Verification items for the finished model (mm, model axes). A direction names the side the tool comes from. Round coordinates to 2 decimals unless told otherwise and drop trailing zeros. Write each loop counter-clockwise with the first axis right and the second up, starting at its lowest first coordinate (ties: lowest second). Pieces come first, ordered by that corner, then holes. Notation, with made-up numbers: M -26.5,31 L -2.5,31 A31 ccw -2.5,61 Z; hole C -29,83.5 d8. An arc over 180 degrees is marked long. One line per question, with ' | ' between items. Start each with the question number.
Q1. Release check for a two-part mould opening along X. For faces 5 (the face through (-8, 0.25, 6)), 6 (the face through (2.8, -0.25, 17.4)), 7 (the face through (-4.124, 3.861, 6.522)), 8 (the face through (4.89, 1.06, 13.24)) record: released by +X, released by -X, zero draft, split by the parting line, or undercut.
Q2. Tool access check on faces 1 (the face through (-6, -3.75, 6)), 2 (the face through (-8, 3.25, 7)), 3 (the face through (-7.874, 2.949, 0.285)), 4 (the face through (-8, -2.4, 6)). Record the directions out of +Z, -Z, +X, -X, +Y, -Y that give a thin tool (end or side, any length) a straight path to the whole face; none if there is none.
Q3. Thickness scan on line 1 along Z through (x, y) = (3.5, 3.1); line 2 along Z through (x, y) = (-6.1, -3); line 3 along X through (y, z) = (-2, 15.7). Record the ranges inside material, lowest first. Write a range as from..to.
Q4. Gauge pin test, flat ends, axial feed: pin 1 (5 mm diameter, centred on x = 6, z = 3, fed in from +Y); pin 2 (5.5 mm diameter, centred on y = 3, z = 17, fed in from -X); pin 3 (0.9 mm diameter, centred on x = 4, z = 15.5, fed in from -Y). Record the tip position at first contact, or that the pin passes through.
Q5. Cross-section at B-B (z = 15). Record the boundary of the cut face in (x, y) (3 decimals).
Q6. Cross-section at C-C (x = -7). Record the boundary of the cut face in (y, z) (3 decimals), then the cut area to 3 significant figures.
Q7. Cross-section at A-A (y = -2). Record the boundary of the cut face in (x, z) (3 decimals).
from build123d import *

# Parameters (mm, degrees)
EXTRUDE002_DEPTH                          = 2.65
EXTRUDE002_ONTO_SKETCH008_ROLL_ANGLE      = 90
EXTRUDE001_DEPTH                          = 2.65
EXTRUDE001_ONTO_SKETCH007_ROLL_ANGLE      = 90
EXTRUDE001_ONTO_SKETCH007_PLACEMENT_ANGLE = 180
EXTRUDE_DEPTH                             = 12.2
SKETCH001_W                               = 12.2
SKETCH001_H                               = 10
PAD_DEPTH                                 = 7
PAD001_DEPTH                              = 12.2
POCKET_DEPTH                              = 19.201
POCKET001_DEPTH                           = 19.201
SKETCH005_R                               = 1.55
POCKET002_DEPTH                           = 7
SKETCH006_R                               = 1.55
POCKET003_DEPTH                           = 7
FILLET_R                                  = 1


with BuildPart() as extrude002:
    # Sketch008 as drawn → Extrude002 (new)
    with BuildSketch(Plane.XY):
        Polygon((3.5, 12.437971), (6.325, 14.068985), (6.325, 19.2), (0.675, 19.2), (0.675, 14.068985), align=None)
    extrude(amount=-EXTRUDE002_DEPTH)


with BuildPart() as extrude002_1:
    # Extrude002 onto Sketch008 roll: moved
    add(extrude002.part.rotate(Axis((0, 0, 0), (1, 0, 0)), EXTRUDE002_ONTO_SKETCH008_ROLL_ANGLE))


with BuildPart() as extrude002_2:
    # Extrude002 onto Sketch008 placement: moved
    add(extrude002_1.part.moved(Location((0, -3.25, 0))))


with BuildPart() as extrude002_3:
    # Extrude002 placement: moved
    add(extrude002_2.part.moved(Location((0, 3, 0))))


with BuildPart() as extrude001:
    # Sketch007 as drawn → Extrude001 (new)
    with BuildSketch(Plane.XY):
        Polygon((2.837971, 6.1), (4.468985, 8.925), (9.6, 8.925), (9.6, 3.275), (4.468985, 3.275), align=None)
    extrude(amount=-EXTRUDE001_DEPTH)


with BuildPart() as extrude001_1:
    # Extrude001 onto Sketch007 roll: moved
    add(extrude001.part.rotate(Axis((0, 0, 0), (1, 0, 0)), EXTRUDE001_ONTO_SKETCH007_ROLL_ANGLE))


with BuildPart() as extrude001_2:
    # Extrude001 onto Sketch007 placement: moved
    add(extrude001_1.part.moved(Location((0, 3.25, 0))).rotate(Axis((0, 3.25, 0), (0, 0, 1)), EXTRUDE001_ONTO_SKETCH007_PLACEMENT_ANGLE))


with BuildPart() as extrude001_3:
    # Extrude001 placement: moved
    add(extrude001_2.part.moved(Location((0, -3, 0))))


with BuildPart() as fillet_body:
    # Sketch → Extrude (new body)
    with BuildSketch(Plane.XY):
        with BuildLine():
            Line((-9.6, -6.75), (-9.6, 3.25))
            Line((-6.1, 3.25), (-9.6, 3.25))
            ThreePointArc((-6.1, 3.25), (-3.625126, 4.275126), (-2.6, 6.75))
            Line((-2.6, 6.75), (9.6, 6.75))
            Line((9.6, 6.75), (9.6, -6.75))
            Line((9.6, -6.75), (-9.6, -6.75))
        make_face()
    extrude(amount=EXTRUDE_DEPTH)

    # Sketch001 → Pad (new body)
    with BuildSketch(Plane.XY.offset(12.2)):
        with Locations((3.5, 1.75)):
            Rectangle(SKETCH001_W, SKETCH001_H)
    extrude(amount=PAD_DEPTH)

    # Sketch002 → Pad001 (new body)
    with BuildSketch(Plane.YZ.offset(9.6)):
        with BuildLine():
            ThreePointArc((-6.75, 12.2), (-4.275126, 13.225126), (-3.25, 15.7))
            Line((-3.25, 12.2), (-3.25, 15.7))
            Line((-6.75, 12.2), (-3.25, 12.2))
        make_face()
    extrude(amount=-PAD001_DEPTH)

    # Sketch003 → Pocket (cut, through all)
    with BuildSketch(Plane.YZ.offset(9.6)):
        with BuildLine():
            Line((6.75, 12.2), (6.75, 0))
            ThreePointArc((6.75, 12.2), (5.383677, 6.1), (6.75, 0))
        make_face()
    extrude(amount=-POCKET_DEPTH, mode=Mode.SUBTRACT)

    # Sketch004 → Pocket001 (cut, through all)
    with BuildSketch(Plane(origin=(0, 0, 0), x_dir=(1, 0, 0), z_dir=(0, 0, -1))):
        with BuildLine():
            Line((-2.6, 6.75), (9.6, 6.75))
            ThreePointArc((-2.6, 6.75), (3.5, 5.383677), (9.6, 6.75))
        make_face()
    extrude(amount=-POCKET001_DEPTH, mode=Mode.SUBTRACT)

    # Sketch005 → Pocket002 (cut, symmetric)
    with BuildSketch(Plane.XZ.offset(3.25)):
        with Locations((3.5, 15.7)):
            Circle(SKETCH005_R)
    extrude(amount=POCKET002_DEPTH, both=True, mode=Mode.SUBTRACT)

    # Sketch006 → Pocket003 (cut, symmetric)
    with BuildSketch(Plane(origin=(0, 3.25, 0), x_dir=(-1, 0, 0), z_dir=(0, 1, 0))):
        with Locations((6.1, 6.1)):
            Circle(SKETCH006_R)
    extrude(amount=POCKET003_DEPTH, both=True, mode=Mode.SUBTRACT)

    # Cut: cut Extrude001
    add(extrude001_3.part, mode=Mode.SUBTRACT)

    # Cut001: cut Extrude002
    add(extrude002_3.part, mode=Mode.SUBTRACT)

    # Fillet
    fillet_edges = [fillet_body.edges().sort_by_distance(p)[0] for p in [
        (-7.85, 3.25, 0),
        (-9.6, -1.75, 0),
        (-6.1, -6.75, 0),
        (3.5, -5.383677, 0),
        (9.6, 0, 0),
        (3.5, 6.75, 0),
        (-3.625126, 4.275126, 0),
    ]]
    fillet(fillet_edges, radius=FILLET_R)


solid = fillet_body.part
Determined:
1) face 5: zero draft | face 6: undercut | face 7: released by -X | face 8: undercut
2) face 1: +Y | face 2: +Z, -Z, -X, +Y | face 3: -Z, -X, +Y | face 4: -X
3) line 1: z = 0..14.15, 17.25..19.2 | line 2: z = 0..4.55, 7.65..12.2 | line 3: x = -2.6..1.95, 5.05..9.6
4) pin 1: stops at y = 6.26 | pin 2: stops at x = -2.6 | pin 3: stops at y = 3.75
5) outline: M -2.6,-3.321 L 2.117,-3.321 L 2.117,-0.25 L 0.675,-0.25 L 0.675,2.4 L 2.117,2.4 L 2.117,3.75 L 4.883,3.75 L 4.883,2.4 L 6.325,2.4 L 6.325,-0.25 L 4.883,-0.25 L 4.883,-3.321 L 9.6,-3.321 L 9.6,6.75 L -2.6,6.75 Z
6) outline: M -6.75,1 A1 ccw -5.75,0 L 2.25,0 A1 ccw 3.25,1 L 3.25,4.838 L 0.25,4.838 L 0.25,3.275 L -2.4,3.275 L -2.4,4.838 L -3.75,4.838 L -3.75,7.362 L -2.4,7.362 L -2.4,8.925 L 0.25,8.925 L 0.25,7.362 L 3.25,7.362 L 3.25,12.2 L -6.75,12.2 Z | area: 95.6 mm²
7) outline: M -9.6,1 A1 ccw -8.6,0 L 8.6,0 A1 ccw 9.6,1 L 9.6,19.2 L -2.6,19.2 L -2.6,12.2 L -9.6,12.2 L -9.6,8.925 L -4.469,8.925 L -2.838,6.1 L -4.469,3.275 L -9.6,3.275 Z; hole C 3.5,15.7 d3.1
